```python
from build123d import *

# Parameters (mm, degrees)
SKETCH1_R           = 12.5
BOSS_EXTRUDE1_DEPTH = 7.5
SKETCH2_W           = 35
SKETCH2_H           = 8.580767914
BOSS_EXTRUDE2_DEPTH = 25
SKETCH3_W           = 25
SKETCH3_H           = 8.580767914
CUT_EXTRUDE1_DEPTH  = 20
SKETCH4_R           = 2.5
BOSS_EXTRUDE3_DEPTH = 3.75
SKETCH5_R           = 2.5
BOSS_EXTRUDE4_DEPTH = 3.75
FILLET2_R           = 2.5
FILLET3_R           = 2.5
CHAMFER1_SIZE       = 5
CHAMFER2_SIZE       = 5


with BuildPart() as part:
    # Sketch1 → Boss-Extrude1 (new body)
    with BuildSketch(Plane(origin=(0, 0, 0), x_dir=(1, 0, 0), z_dir=(0, 1, 0))):
        Circle(SKETCH1_R)
    extrude(amount=BOSS_EXTRUDE1_DEPTH)

    # Sketch2 → Boss-Extrude2 (add)
    with BuildSketch(Plane(origin=(0, 7.5, 0), x_dir=(1, 0, 0), z_dir=(0, 1, 0))):
        Rectangle(SKETCH2_W, SKETCH2_H)
    extrude(amount=BOSS_EXTRUDE2_DEPTH)

    # Sketch3 → Cut-Extrude1 (cut)
    with BuildSketch(Plane(origin=(0, 32.5, 0), x_dir=(1, 0, 0), z_dir=(0, 1, 0))):
        Rectangle(SKETCH3_W, SKETCH3_H)
    extrude(amount=-CUT_EXTRUDE1_DEPTH, mode=Mode.SUBTRACT)

    # Sketch4 → Boss-Extrude3 (add)
    with BuildSketch(Plane(origin=(-12.5, 0, 0), x_dir=(0, 0, -1), z_dir=(1, 0, 0))):
        with Locations((0, 27.5)):
            Circle(SKETCH4_R)
    extrude(amount=BOSS_EXTRUDE3_DEPTH)

    # Sketch5 → Boss-Extrude4 (add)
    with BuildSketch(Plane.ZY.offset(-12.5)):
        with Locations((0, 27.5)):
            Circle(SKETCH5_R)
    extrude(amount=BOSS_EXTRUDE4_DEPTH)

    # Fillet2
    fillet2_edges = [part.edges().sort_by_distance(p)[0] for p in [
        (-8.75, 27.5, 2.5),
    ]]
    fillet(fillet2_edges, radius=FILLET2_R)

    # Fillet3
    fillet3_edges = [part.edges().sort_by_distance(p)[0] for p in [
        (8.75, 27.5, -2.5),
    ]]
    fillet(fillet3_edges, radius=FILLET3_R)

    # Chamfer1
    chamfer1_edges = [part.edges().sort_by_distance(p)[0] for p in [
        (-12.5, 12.5, 0),
    ]]
    chamfer(chamfer1_edges, length=CHAMFER1_SIZE)

    # Chamfer2
    chamfer2_edges = [part.edges().sort_by_distance(p)[0] for p in [
        (12.5, 12.5, 0),
    ]]
    chamfer(chamfer2_edges, length=CHAMFER2_SIZE)


solid = part.part
```
Can you work these out from the model? Positions are in its coordinate system, mm. A direction names the side the tool comes from. Round coordinates to 2 decimals unless told otherwise and drop trailing zeros. Order: outer loops, then holes, each group sorted by start corner. A loop starts at its lowest first (then second) coordinate and runs counter-clockwise, first axis right, second up.
(1) If we section it at B-B (z = 0): Please give me the cut outline in (x, y), plus the area to 3 significant figures.
Results are:
outline: (-17.5, 7.5) - (-12.5, 7.5) - (-12.5, 0) - (12.5, 0) - (12.5, 7.5) - (17.5, 7.5) - (17.5, 32.5) - (12.5, 32.5) - (12.5, 30) - (11.25, 30) arc R2.5 ccw to (11.25, 25) - (12.5, 25) - (12.5, 17.5) - (7.5, 12.5) - (-7.5, 12.5) - (-12.5, 17.5) - (-12.5, 25) - (-11.25, 25) arc R2.5 ccw to (-11.25, 30) - (-12.5, 30) - (-12.5, 32.5) - (-17.5, 32.5) - close
area: 620 mm2
(2) If I drill on L1, parallel to X at y = 19.5, z = 3; L2, parallel to Z at x = 1, y = 11; L3, parallel to Y at x = 7.5, z = 9.25, over which ranges is the centre line in solid material (lowest first)?
Results are:
L1: x = -17.5 to -12.5, 12.5 to 17.5
L2: z = -4.29 to 4.29
L3: y = 0 to 7.5
(3) We'd pull the mould along X, two halves only. Please class faces 6 (the face through (-15, 32.5, 0)), 7 (the face through (17.5, 20, 0)), 8 (the face through (-10, 15, 0)): +X half, -X half, draft (parallel to the pull), parting line (faces both ways), or undercut.
Results are:
face 6: draft
face 7: +X half
face 8: undercut
(4) If we section it at A-A (y = 22): Please give me the cut outline in (x, z), plus the area to 3 significant figures.
Results are:
outline: (-17.5, -4.29) - (-12.5, -4.29) - (-12.5, 4.29) - (-17.5, 4.29) - close; (12.5, -4.29) - (17.5, -4.29) - (17.5, 4.29) - (12.5, 4.29) - close
area: 85.8 mm2
(5) I'm going to push flat-ended pins straight in: pin 1 (12.5 mm diameter, centred on x = -7.5, y = 26, fed in from +Z); pin 2 (4.5 mm diameter, centred on x = 0.5, z = 0.5, fed in from +Y); pin 3 (2 mm diameter, centred on x = 6, y = 11, fed in from -Z). Where does each tip first touch, or does it pass through?
Results are:
pin 1: stops at z = 4.29
pin 2: stops at y = 12.5
pin 3: stops at z = -4.29
(6) If we section it at D-D (x = 10): Please give me the cut outline in (y, z).
Results are:
outline: (0, -7.5) - (7.5, -7.5) - (7.5, -4.29) - (15, -4.29) - (15, 4.29) - (7.5, 4.29) - (7.5, 7.5) - (0, 7.5) - close; circle Ø4.33 at (27.5, 0)
(7) If we section it at C-C (x = 0): Please give me the cut outline in (y, z), plus the area to 3 significant figures.
Results are:
outline: (0, -12.5) - (7.5, -12.5) - (7.5, -4.29) - (12.5, -4.29) - (12.5, 4.29) - (7.5, 4.29) - (7.5, 12.5) - (0, 12.5) - close
area: 230 mm2
(8) On a 3-axis mill with a long thin cutter (end or side, diameter ignored), from which of +Z, -Z, +X, -X, +Y, -Y can I reach the whole of each face in a straight line? I mean faces 1 (the face through (0, 7.5, -8)), 2 (the face through (0, 12.5, 0)), 3 (the face through (12, 30, 0)), 4 (the face through (11.923, 3.698, -3.755)), 5 (the face through (0, 7.5, 7)). Say none if no direction works.
Results are:
face 1: -Z, +X, -X, +Y
face 2: +Z, -Z, +Y
face 3: none
face 4: -Y
face 5: +Z, +X, -X, +Y
